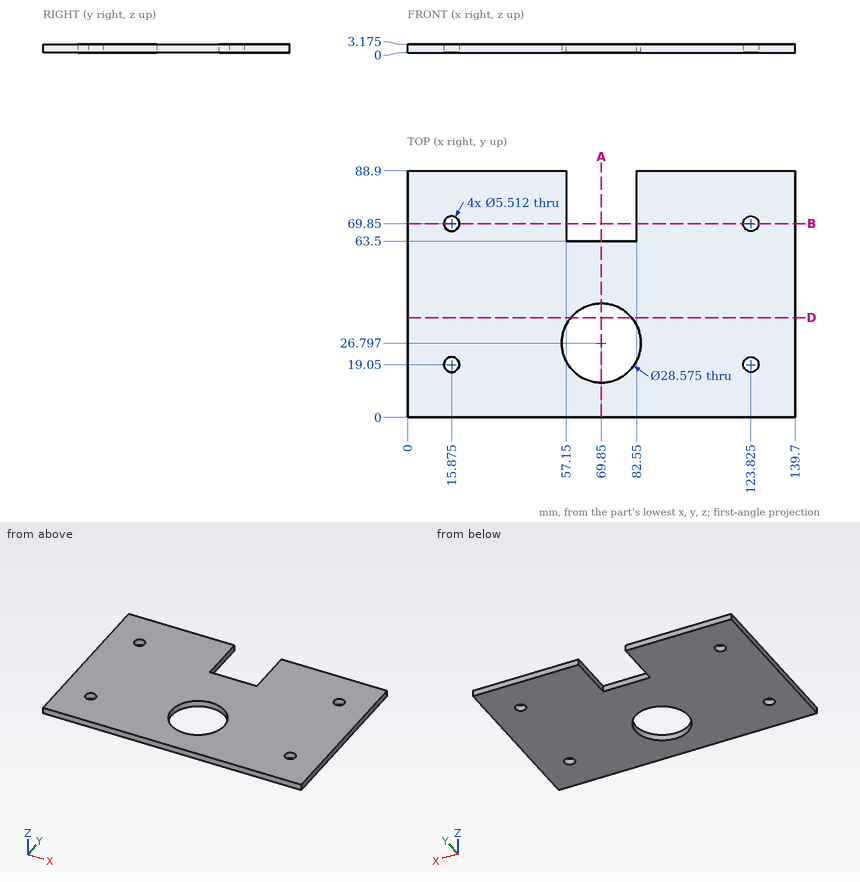
Input: dimensioned drawing with shaded views. Units: mm. Origin: part minimum x, y, z. Give positions to 0.01 mm unless a question says otherwise; leave off trailing zeros. Write each loop counter-clockwise with the first axis right and the second up, starting at its lowest first coordinate (ties: lowest second). Pieces come first, ordered by that corner, then holes.
1. Section query D-D, the plane y = 36. Return loops of the section in (x, z) (1 decimal), then the cut area to 3 significant figures.
2. Line query: probe 1 along X at (y, z) = (69.85, 2.1); probe 2 along Y at (x, z) = (15.5, 0.25); probe 3 along Y at (x, z) = (69.85, 1.4). Output: solid intervals per line, ascending.
3. Section query B-B, the plane y = 69.85. Count the separate pieces of the cut face and the enclosed holes in it, then the cut area to 3 significant figures.
4. Section query A-A, the plane x = 69.85. Return loops of the section in (y, z) (1 decimal).
5. Pin query (flat end, axial travel): P1, Ø1.5, axis at x = 69.5, z = 2.5, coming from the +Y side. Return the tip coordinate at first contact, or that it passes through.
Computed:
1. outline: (0, 0) - (58.9, 0) - (58.9, 3.2) - (0, 3.2) - close; (80.8, 0) - (139.7, 0) - (139.7, 3.2) - (80.8, 3.2) - close
1. area: 374 mm2
2. probe 1: x = 0 to 13.12, 18.63 to 57.15, 82.55 to 121.07, 126.58 to 139.7
2. probe 2: y = 0 to 16.32, 21.78 to 67.12, 72.58 to 88.9
2. probe 3: y = 0 to 12.51, 41.08 to 63.5
3. separate pieces: 4
3. enclosed holes: 0
3. area: 328 mm2
4. outline: (0, 0) - (12.5, 0) - (12.5, 3.2) - (0, 3.2) - close; (41.1, 0) - (63.5, 0) - (63.5, 3.2) - (41.1, 3.2) - close
5. P1: stops at y = 63.5
